Verification items for the finished model (mm, model axes). A direction names the side the tool comes from. Coordinates: 2 decimals unless noted, no trailing zeros. Write each loop counter-clockwise with the first axis right and the second up, starting at its lowest first coordinate (ties: lowest second). Pieces come first, ordered by that corner, then holes. Notation, with made-up numbers: (6, 59.5) -> (20, 59.5) arc R15 cw to (20, 72.5) -> close; hole circle Ø7 at (-18, 23). An arc over 180 degrees is marked (long way). Use CSV: the item, a comma, the result in double quotes.
```python
from build123d import *

# Parameters (mm, degrees)
BOSS_EXTRUDE3_DEPTH = 27
SKETCH7_R           = 1.35
CUT_EXTRUDE2_DEPTH  = 20
SKETCH8_R           = 1
CUT_EXTRUDE3_DEPTH  = 20


with BuildPart() as part:
    # Sketch5 → Boss-Extrude3 (new body)
    with BuildSketch(Plane.XY):
        Polygon((0, 0), (-30, 0), (-34.331775419, -17.903100957), (-32.399923767, -18.420739047), (-28, -2), (0, -2), align=None)
    extrude(amount=BOSS_EXTRUDE3_DEPTH)

    # Sketch7 → Cut-Extrude2 (cut)
    with BuildSketch(Plane(origin=(0, 0, 0), x_dir=(1, 0, 0), z_dir=(0, 1, 0))):
        with Locations(Location((-17.22649731, -5.5, 0), (0, 0, 270))):
            Circle(SKETCH7_R)
        with Locations(Location((-17.22649731, -9.5, 0), (0, 0, 270))):
            Circle(SKETCH7_R)
        with Locations(Location((-5.22649731, -5.5, 0), (0, 0, 270))):
            Circle(SKETCH7_R)
        with Locations(Location((-5.22649731, -9.5, 0), (0, 0, 270))):
            Circle(SKETCH7_R)
        with Locations(Location((-5.22649731, -17.5, 0), (0, 0, 180))):
            Circle(SKETCH7_R)
        with Locations(Location((-5.22649731, -21.5, 0), (0, 0, 180))):
            Circle(SKETCH7_R)
        with Locations(Location((-17.22649731, -17.5, 0), (0, 0, 180))):
            Circle(SKETCH7_R)
        with Locations(Location((-17.22649731, -21.5, 0), (0, 0, 180))):
            Circle(SKETCH7_R)
    extrude(amount=-CUT_EXTRUDE2_DEPTH, mode=Mode.SUBTRACT)

    # Sketch8 → Cut-Extrude3 (cut)
    with BuildSketch(Plane(origin=(-28.340840747, 6.857256606, 0), x_dir=(0, 0, 1), z_dir=(-0.9719540583604048, 0.23517080693984682, 0))):
        with Locations(Location((3, -10.855124208, 0), (0, 0, 270))):
            Circle(SKETCH8_R)
        with Locations(Location((3, -23.155124208, 0), (0, 0, 270))):
            Circle(SKETCH8_R)
        with Locations(Location((24, -23.155124208, 0), (0, 0, 270))):
            Circle(SKETCH8_R)
        with Locations(Location((24, -10.855124208, 0), (0, 0, 270))):
            Circle(SKETCH8_R)
    extrude(amount=-CUT_EXTRUDE3_DEPTH, mode=Mode.SUBTRACT)


solid = part.part
```
1) Set-up check for faces 1 (the flat face through (-14, -2, 13)), 2 (the flat face through (0, -1, 13)): record each of +Z, -Z, +X, -X, +Y, -Y from which the full face is reachable in a straight line by a thin tool's end or side.
Return value:
face 1,"+Z, -Z, +X, -Y"
face 2,"+Z, -Z, +X, +Y, -Y"
2) Cross-section at B-B (z = 12.5). Record the boundary of the cut face in (x, y).
Return value:
outline,"(-34.33, -17.9) -> (-32.4, -18.42) -> (-28, -2) -> (0, -2) -> (0, 0) -> (-30, 0) -> close"
3) Gauge pin test, flat ends, axial feed: pin 1 (2.5 mm diameter, centred on x = -5.23, z = 9.5, fed in from +Y); pin 2 (2 mm diameter, centred on x = -26, z = 10.5, fed in from -Y); pin 3 (3 mm diameter, centred on x = -5.23, z = 5.5, fed in from +Y); pin 4 (1 mm diameter, centred on y = -12, z = 8.5, fed in from +X). Record the tip position at first contact, or that the pin passes through.
Return value:
pin 1,"through"
pin 2,"y = -2"
pin 3,"y = 0"
pin 4,"x = -30.55"
4) Scan lines: L1, parallel to X at y = -0.7, z = 5.5; L2, parallel to X at y = -0.4, z = 5.5; L3, parallel to Y at x = -1.5, z = 4.25. Record each from-to range of solid material in increasing order.
Return value:
L1,"-30.17 to -18.58, -15.88 to -6.58, -3.88 to 0"
L2,"-30.1 to -18.58, -15.88 to -6.58, -3.88 to 0"
L3,"-2 to 0"
5) Cross-section at A-A (z = 9.5). Record the boundary of the cut face in (x, y).
Return value:
outline,"(-34.33, -17.9) -> (-32.4, -18.42) -> (-28, -2) -> (-18.58, -2) -> (-18.58, 0) -> (-30, 0) -> close; (-15.88, -2) -> (-6.58, -2) -> (-6.58, 0) -> (-15.88, 0) -> close; (-3.88, -2) -> (0, -2) -> (0, 0) -> (-3.88, 0) -> close"
6) Cross-section at C-C (y = -4.25). Give the number of separate pieces and of enclosed holes in the cut face, plus the area to 3 significant figures.
Return value:
separate pieces,"3"
enclosed holes,"0"
area,"56.3 mm2"
7) Mould release check, pull along Z, two halves, no side actions. Record for faces 3 (the flat face through (-21.1, -1.7, 27)), 4 (the flat face through (-33.38, -18.16, 13.31)), 5 (the cylindrical face through (-16.821, -0.986, 6.788)): released by +Z, released by -Z, zero draft, split by the parting line, or undercut.
Return value:
face 3,"released by +Z"
face 4,"zero draft"
face 5,"undercut"
8) Cross-section at D-D (z = 23.5). Record the boundary of the cut face in (x, y).
Return value:
outline,"(-34.33, -17.9) -> (-32.4, -18.42) -> (-32.01, -16.97) -> (-33.99, -16.49) -> close; (-33.58, -14.81) -> (-31.56, -15.3) -> (-28.83, -5.08) -> (-31.1, -4.54) -> close; (-30.69, -2.85) -> (-28.38, -3.41) -> (-28, -2) -> (0, -2) -> (0, 0) -> (-30, 0) -> close"
